Work out the finished part from the listing and answer in its coordinate system (mm). Give positions to 0.01 mm unless a question says otherwise; leave off trailing zeros. Order: outer loops, then holes, each group sorted by start corner. A loop starts at its lowest first (then second) coordinate and runs counter-clockwise, first axis right, second up.
```python
from build123d import *

# Parameters (mm, degrees)
BASE_DEPTH                 = 5
F_3_2_3_2_DIAMETER_HOLE1_D = 3.2


with BuildPart() as part:
    # Sketch1 → base (new, symmetric)
    with BuildSketch(Plane(origin=(0, 0, 0), x_dir=(1, 0, 0), z_dir=(0, 1, 0))):
        with BuildLine():
            Line((-155.395037554, 141.25290193), (-162.473770491, 148.331634867))
            ThreePointArc((-162.473770491, 148.331634867), (-203.253497152, 84.19035512), (-219.772609758, 10))
            Line((-219.772609758, 10), (-209.761769634, 10))
            ThreePointArc((-209.761769634, 10), (-194.014701827, 80.363520797), (-155.395037554, 141.25290193))
        make_face()
    extrude(amount=BASE_DEPTH, both=True)

    # Ø3.2 (3.2) Diameter Hole1 (through all)
    with Locations(Plane(origin=(0, 5, 0), x_dir=(1, 0, 0), z_dir=(0, 1, 0))):
        with Locations((-164.699555271, 138.199336083), (-214.18186009, 18.738484691)):
            Hole(F_3_2_3_2_DIAMETER_HOLE1_D / 2)


solid = part.part
```
1. The part is cut by section A-A (x = -164.5). Write down the section's boundary in (y, z), then the cut area to 3 significant figures.
Findings below:
outline: (-5, -146.08) - (5, -146.08) - (5, -139.79) - (-5, -139.79) - close; (-5, -136.61) - (5, -136.61) - (5, -130.54) - (-5, -130.54) - close
area: 124 mm2
2. The part is cut by section C-C (x = -214.5). Write down the section's boundary in (y, z), then the cut area to 3 significant figures.
Findings below:
outline: (-5, -48.89) - (5, -48.89) - (5, -20.31) - (-5, -20.31) - close; (-5, -17.17) - (5, -17.17) - (5, -10) - (-5, -10) - close
area: 357 mm2
3. Straight lines are drawn through the part: probe 1 along Z at (x, y) = (-163.5, -1.5); probe 2 along X at (y, z) = (4, -108); probe 3 along Z at (x, y) = (-160, 2). For each, find the intervals that lie inside material, in ascending order.
Findings below:
probe 1: z = -147.2 to -139.26, -137.14 to -131.79
probe 2: x = -191.67 to -180.1
probe 3: z = -145.86 to -136.01
4. The part is cut by section D-D (z = -108.5). Write down the section's boundary in (x, y), then the cut area to 3 significant figures.
Findings below:
outline: (-191.38, -5) - (-179.8, -5) - (-179.8, 5) - (-191.38, 5) - close
area: 116 mm2
5. The part is cut by section B-B (y = 0.75). Write down the section's boundary in (x, z), then the cut area to 3 significant figures.
Findings below:
outline: (-219.77, -10) arc R220 ccw to (-162.47, -148.33) - (-155.4, -141.25) arc R210 cw to (-209.76, -10) - close; hole circle Ø3.2 at (-214.18, -18.74); hole circle Ø3.2 at (-164.7, -138.2)
area: 1,470 mm2
6. The mould has two halves that part along Z. Classify faces 1 (the face through (-158.88, 0.07, -144.74)), 2 (the face through (-163.52, -0.07, -139.28)), 3 (the face through (-194.4, 0.07, -79.43)): pulls with the +Z half, pulls with the -Z half, needs draft (parallel to the pull), parting line crosses it, or undercut.
Findings below:
face 1: pulls with the -Z half
face 2: undercut
face 3: pulls with the +Z half
7. Given P1, Ø3, axis at y = 3.5, z = -115.5, coming from the -X side; P2, Ø2, axis at x = -165.5, y = -2.5, coming from the +Z side; P3, Ø1, axis at x = -204, y = 0.5, coming from the -Z side, each flat-ended and moving along its own axis, determine where each tip first touches the part or whether it passes through.
Findings below:
P1: stops at x = -188.16
P2: stops at z = -127.98
P3: stops at z = -83.59
